from build123d import *

# Parameters (mm, degrees)
BOSS_EXTRUDE1_DEPTH                           = 15.875
BOSS_EXTRUDE2_DEPTH                           = 15.875
CBORE_FOR_1_4_SOCKET_HEAD_CAP_SCREW1_AT_COUNT = 2
CBORE_FOR_1_4_SOCKET_HEAD_CAP_SCREW1_AT_PITCH = 41.275
MOVE_FACE1_BY                                 = 0.127
MOVE_FACE1_2_BY                               = 0.127
MOVE_START                                    = 28.575
MOVE_FACE2_OUTLINE_W                          = 15.875
MOVE_FACE2_OUTLINE_H                          = 60.325
MOVE_FACE2_OUTLINE_R                          = 5.55625
MOVE_FACE2_DEPTH                              = 6.35
MOVE_START_2                                  = 22.225
MOVE_FACE2_2_OUTLINE_R                        = 5.55625
MOVE_FACE2_2_OUTLINE_R_2                      = 3.57124
MOVE_FACE2_2_DEPTH                            = 6.35


with BuildPart() as part:
    # Sketch1 → Boss-Extrude1 (new body)
    with BuildSketch(Plane(origin=(0, 0, 0), x_dir=(0, 0, -1), z_dir=(1, 0, 0))):
        with BuildLine():
            Line((30.1625, 0), (14.2875, 0))
            ThreePointArc((14.2875, 0), (0, -14.2875), (-14.2875, 0))
            Line((-14.2875, 0), (-30.1625, 0))
            Line((-30.1625, 0), (-30.1625, -34.925))
            Line((-30.1625, -34.925), (30.1625, -34.925))
            Line((30.1625, -34.925), (30.1625, 0))
        make_face()
    extrude(amount=BOSS_EXTRUDE1_DEPTH)


with BuildPart() as body_2:
    # Sketch1<3> → Boss-Extrude2 (new body)
    with BuildSketch(Plane(origin=(0, 0, 0), x_dir=(0, 0, -1), z_dir=(1, 0, 0))):
        with BuildLine():
            ThreePointArc((-14.2875, 0), (0, 14.2875), (14.2875, 0))
            Line((14.2875, 0), (30.1625, 0))
            Line((30.1625, 0), (30.1625, 34.925))
            Line((30.1625, 34.925), (-30.1625, 34.925))
            Line((-30.1625, 34.925), (-30.1625, 0))
            Line((-30.1625, 0), (-14.2875, 0))
        make_face()
    extrude(amount=BOSS_EXTRUDE2_DEPTH)


with BuildPart() as cbore_for_1_4_socket_head_cap_screw1_tool:
    # Sketch4 → CBORE for 1/4 Socket Head Cap Screw1 (revolve)
    with BuildSketch(Plane(origin=(7.9375, 34.925, 20.6375), x_dir=(0, 0, 1), z_dir=(1, 0, 0))):
        Polygon((0, 0), (0, 69.85), (3.57124, 69.85), (3.57124, 6.35), (5.55625, 6.35), (5.55625, 0.635), (6.19125, 0), align=None)
    cbore_for_1_4_socket_head_cap_screw1 = revolve(axis=Axis((7.9375, 41.275, 20.6375), (0, -1, 0)))


with BuildPart() as part_1:
    add(part.part)

    # CBORE for 1/4 Socket Head Cap Screw1: cut by cbore_for_1_4_socket_head_cap_screw1_tool
    add(cbore_for_1_4_socket_head_cap_screw1_tool.part, mode=Mode.SUBTRACT)


with BuildPart() as body_2_1:
    add(body_2.part)

    # CBORE for 1/4 Socket Head Cap Screw1: cut by cbore_for_1_4_socket_head_cap_screw1_tool
    add(cbore_for_1_4_socket_head_cap_screw1_tool.part, mode=Mode.SUBTRACT)


with BuildPart() as cbore_for_1_4_socket_head_cap_screw1_at_tool:
    # CBORE for 1/4 Socket Head Cap Screw1 at: CBORE for 1/4 Socket Head Cap Screw1 ×2
    with Locations(*[(0, 0, -i * CBORE_FOR_1_4_SOCKET_HEAD_CAP_SCREW1_AT_PITCH) for i in range(1, CBORE_FOR_1_4_SOCKET_HEAD_CAP_SCREW1_AT_COUNT)]):
        add(cbore_for_1_4_socket_head_cap_screw1)


with BuildPart() as part_2:
    add(part_1.part)

    # CBORE for 1/4 Socket Head Cap Screw1 at: cut by cbore_for_1_4_socket_head_cap_screw1_at_tool
    add(cbore_for_1_4_socket_head_cap_screw1_at_tool.part, mode=Mode.SUBTRACT)

    # Move Face1 2: a curved face moved inward by 0.127
    add(Solid.thicken(part_2.faces().sort_by_distance((7.9375, -14.2875, 0))[0], -MOVE_FACE1_2_BY), mode=Mode.SUBTRACT)

    # Chamfer2
    # the kernel refuses this chamfer: 0.635 mm, written as the material it takes off along each edge
    with BuildSketch(Plane(origin=(0, 0, 0), x_dir=(0, 0.1132288377802066, -0.9935689358544497), z_dir=(0, 0.9935689358544497, 0.1132288377802066))) as chamfer2_piece_1:
        with BuildLine():
            Line((15.067460512, 0.017960512), (14.396539488, -0.652960512))
            Line((14.396539488, -0.652960512), (14.383839488, -0.652960512))
            ThreePointArc((14.383839488, -0.652960512), (14.4018, -0.326480256), (14.4018, 0))
            Line((14.4018, 0), (14.4145, 0.0127))
            ThreePointArc((14.4145, 0.0127), (14.740980256, 0.0127), (15.067460512, 0.030660512))
            Line((15.067460512, 0.030660512), (15.067460512, 0.017960512))
        make_face()
    revolve(axis=Axis((0, 0, 0), (-1, 0, 0)), revolution_arc=193.002955297, mode=Mode.SUBTRACT)
    with BuildSketch(Plane(origin=(-1.600435701, 0, -14.4145), x_dir=(0, 0, -1), z_dir=(1, 0, 0))) as chamfer2_piece_2:
        with BuildLine():
            Line((0.639932919, 0.017577515), (-0.031172593, -0.625784266))
            Line((-0.031172593, -0.625784266), (-0.043861283, -0.625248401))
            ThreePointArc((-0.043861283, -0.625248401), (-0.016099091, -0.31288099), (-0.0127, 0))
            Line((-0.0127, 0), (0, 0.0127))
            ThreePointArc((0, 0.0127), (0.319966459, 0.0127), (0.639932919, 0.030277515))
            Line((0.639932919, 0.030277515), (0.639932919, 0.017577515))
        make_face()
    extrude(amount=19.075871403, mode=Mode.SUBTRACT)
    with BuildSketch(Plane(origin=(-1.600435701, 0, 14.4145), x_dir=(0, -0.999777333387341, -0.021101745067597762), z_dir=(1, 0, 0))) as chamfer2_piece_3:
        with BuildLine():
            Line((0.626302721, 0.017960512), (-0.031077302, -0.639419511))
            Line((-0.031077302, -0.639419511), (-0.043774474, -0.639151519))
            ThreePointArc((-0.043774474, -0.639151519), (-0.019449023, -0.319627221), (-0.012697172, 0.000267992))
            Line((-0.012697172, 0.000267992), (0.000267992, 0.012697172))
            ThreePointArc((0.000267992, 0.012697172), (0.313151041, 0.009493172), (0.626034729, 0.030657684))
            Line((0.626034729, 0.030657684), (0.626302721, 0.017960512))
        make_face()
    extrude(amount=19.075871403, mode=Mode.SUBTRACT)
    with BuildSketch(Plane(origin=(15.875, 0, 0), x_dir=(0, 0.11322883778020662, -0.9935689358544497), z_dir=(0, 0.9935689358544497, 0.11322883778020662))) as chamfer2_piece_4:
        with BuildLine():
            Line((14.396539488, 0.652960512), (15.067460512, -0.017960512))
            Line((15.067460512, -0.017960512), (15.067460512, -0.030660512))
            ThreePointArc((15.067460512, -0.030660512), (14.740980256, -0.0127), (14.4145, -0.0127))
            Line((14.4145, -0.0127), (14.4018, 0))
            ThreePointArc((14.4018, 0), (14.4018, 0.326480256), (14.383839488, 0.652960512))
            Line((14.383839488, 0.652960512), (14.396539488, 0.652960512))
        make_face()
    revolve(axis=Axis((15.875, 0, 0), (-1, 0, 0)), revolution_arc=193.002955297, mode=Mode.SUBTRACT)


with BuildPart() as body_2_2:
    add(body_2_1.part)

    # CBORE for 1/4 Socket Head Cap Screw1 at: cut by cbore_for_1_4_socket_head_cap_screw1_at_tool
    add(cbore_for_1_4_socket_head_cap_screw1_at_tool.part, mode=Mode.SUBTRACT)

    # Move Face1: a curved face moved inward by 0.127
    add(Solid.thicken(body_2_2.faces().sort_by_distance((7.9375, 14.2875, 0))[0], -MOVE_FACE1_BY), mode=Mode.SUBTRACT)

    # Move Face2: read off the stored shape, not the designer's step
    # Move Face2 outline → Move Face2 (cut)
    with BuildSketch(Plane(origin=(0, 0, 0), x_dir=(1, 0, 0), z_dir=(0, 1, 0)).offset(MOVE_START)):
        with Locations((7.9375, 0)):
            Rectangle(MOVE_FACE2_OUTLINE_W, MOVE_FACE2_OUTLINE_H)
        with Locations((7.9375, -20.6375)):
            Circle(MOVE_FACE2_OUTLINE_R, mode=Mode.SUBTRACT)
        with Locations((7.9375, 20.6375)):
            Circle(MOVE_FACE2_OUTLINE_R, mode=Mode.SUBTRACT)
    extrude(amount=MOVE_FACE2_DEPTH, mode=Mode.SUBTRACT)

    # Move Face2 2 outline → Move Face2 2 (cut)
    # profile 1 of 2: a face of its own
    with BuildSketch(Plane(origin=(0, 0, 0), x_dir=(1, 0, 0), z_dir=(0, 1, 0)).offset(MOVE_START_2)):
        with Locations((7.9375, 20.6375)):
            Circle(MOVE_FACE2_2_OUTLINE_R)
        with Locations((7.9375, 20.6375)):
            Circle(MOVE_FACE2_2_OUTLINE_R_2, mode=Mode.SUBTRACT)
    # profile 2 of 2: a face of its own
    with BuildSketch(Plane(origin=(0, 0, 0), x_dir=(1, 0, 0), z_dir=(0, 1, 0)).offset(MOVE_START_2)):
        with Locations((7.9375, -20.6375)):
            Circle(MOVE_FACE2_2_OUTLINE_R)
        with Locations((7.9375, -20.6375)):
            Circle(MOVE_FACE2_2_OUTLINE_R_2, mode=Mode.SUBTRACT)
    extrude(amount=MOVE_FACE2_2_DEPTH, mode=Mode.SUBTRACT)

    # Move Face2 3: loft between two sections, ruled curve by curve
    move_face2_3_from = [
        Edge.make_three_point_arc((7.9375, 27.94, -15.08125), (13.49375, 27.94, -20.6375), (7.9375, 27.94, -26.19375)),
        Edge.make_three_point_arc((7.9375, 27.94, -26.19375), (2.38125, 27.94, -20.6375), (7.9375, 27.94, -15.08125)),
    ]
    move_face2_3_to = [
        Edge.make_three_point_arc((7.9375, 28.575, -14.44625), (14.12875, 28.575, -20.6375), (7.9375, 28.575, -26.82875)),
        Edge.make_three_point_arc((7.9375, 28.575, -26.82875), (1.74625, 28.575, -20.6375), (7.9375, 28.575, -14.44625)),
    ]
    move_face2_3 = Solid(Shell([*[Face.make_surface_from_curves(move_face2_3_from[k], move_face2_3_to[k]) for k in range(2)], Face(Wire(move_face2_3_from)), Face(Wire(move_face2_3_to))]))
    add(move_face2_3, mode=Mode.SUBTRACT)

    # Move Face2 4: loft between two sections, ruled curve by curve
    move_face2_4_from = [
        Edge.make_three_point_arc((7.9375, 27.94, 26.19375), (13.49375, 27.94, 20.6375), (7.9375, 27.94, 15.08125)),
        Edge.make_three_point_arc((7.9375, 27.94, 15.08125), (2.38125, 27.94, 20.6375), (7.9375, 27.94, 26.19375)),
    ]
    move_face2_4_to = [
        Edge.make_three_point_arc((7.9375, 28.575, 26.82875), (14.12875, 28.575, 20.6375), (7.9375, 28.575, 14.44625)),
        Edge.make_three_point_arc((7.9375, 28.575, 14.44625), (1.74625, 28.575, 20.6375), (7.9375, 28.575, 26.82875)),
    ]
    move_face2_4 = Solid(Shell([*[Face.make_surface_from_curves(move_face2_4_from[k], move_face2_4_to[k]) for k in range(2)], Face(Wire(move_face2_4_from)), Face(Wire(move_face2_4_to))]))
    add(move_face2_4, mode=Mode.SUBTRACT)

    # Chamfer1
    # the kernel refuses this chamfer: 0.635 mm, written as the material it takes off along each edge
    with BuildSketch(Plane(origin=(0, 0, 0), x_dir=(0, -0.11322883778020673, 0.9935689358544497), z_dir=(0, -0.9935689358544497, -0.11322883778020673))) as chamfer1_piece_1:
        with BuildLine():
            Line((15.067460512, 0.017960512), (14.396539488, -0.652960512))
            Line((14.396539488, -0.652960512), (14.383839488, -0.652960512))
            ThreePointArc((14.383839488, -0.652960512), (14.4018, -0.326480256), (14.4018, 0))
            Line((14.4018, 0), (14.4145, 0.0127))
            ThreePointArc((14.4145, 0.0127), (14.740980256, 0.0127), (15.067460512, 0.030660512))
            Line((15.067460512, 0.030660512), (15.067460512, 0.017960512))
        make_face()
    revolve(axis=Axis((0, 0, 0), (-1, 0, 0)), revolution_arc=193.002955297, mode=Mode.SUBTRACT)
    with BuildSketch(Plane(origin=(-1.600435701, 0, 14.4145), x_dir=(0, 0, 1), z_dir=(1, 0, 0))) as chamfer1_piece_2:
        with BuildLine():
            Line((0.639932919, 0.017577515), (-0.031172593, -0.625784266))
            Line((-0.031172593, -0.625784266), (-0.043861283, -0.625248401))
            ThreePointArc((-0.043861283, -0.625248401), (-0.016099091, -0.31288099), (-0.0127, 0))
            Line((-0.0127, 0), (0, 0.0127))
            ThreePointArc((0, 0.0127), (0.319966459, 0.0127), (0.639932919, 0.030277515))
            Line((0.639932919, 0.030277515), (0.639932919, 0.017577515))
        make_face()
    extrude(amount=19.075871403, mode=Mode.SUBTRACT)
    with BuildSketch(Plane(origin=(-1.600435701, 0, -14.4145), x_dir=(0, 0.999777333387341, 0.021101745067597762), z_dir=(1, 0, 0))) as chamfer1_piece_3:
        with BuildLine():
            Line((0.626302721, 0.017960512), (-0.031077302, -0.639419511))
            Line((-0.031077302, -0.639419511), (-0.043774474, -0.639151519))
            ThreePointArc((-0.043774474, -0.639151519), (-0.019449023, -0.319627221), (-0.012697172, 0.000267992))
            Line((-0.012697172, 0.000267992), (0.000267992, 0.012697172))
            ThreePointArc((0.000267992, 0.012697172), (0.313151041, 0.009493172), (0.626034729, 0.030657684))
            Line((0.626034729, 0.030657684), (0.626302721, 0.017960512))
        make_face()
    extrude(amount=19.075871403, mode=Mode.SUBTRACT)
    with BuildSketch(Plane(origin=(15.875, 0, 0), x_dir=(0, -0.11322883778020675, 0.9935689358544497), z_dir=(0, -0.9935689358544497, -0.11322883778020675))) as chamfer1_piece_4:
        with BuildLine():
            Line((14.396539488, 0.652960512), (15.067460512, -0.017960512))
            Line((15.067460512, -0.017960512), (15.067460512, -0.030660512))
            ThreePointArc((15.067460512, -0.030660512), (14.740980256, -0.0127), (14.4145, -0.0127))
            Line((14.4145, -0.0127), (14.4018, 0))
            ThreePointArc((14.4018, 0), (14.4018, 0.326480256), (14.383839488, 0.652960512))
            Line((14.383839488, 0.652960512), (14.396539488, 0.652960512))
        make_face()
    revolve(axis=Axis((15.875, 0, 0), (-1, 0, 0)), revolution_arc=193.002955297, mode=Mode.SUBTRACT)


solid = body_2_2.part
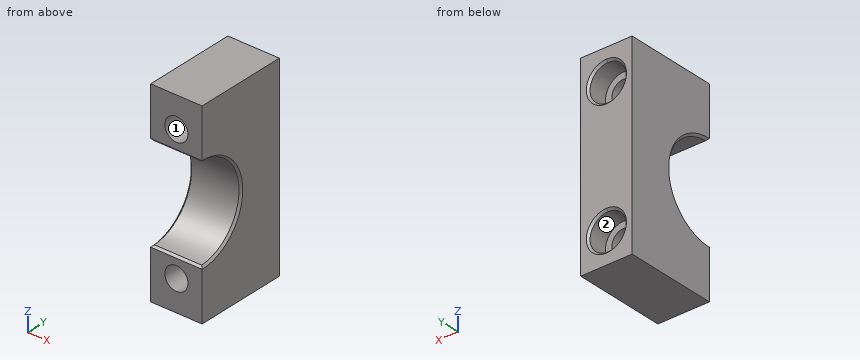
Geometry: final body of the model. Coordinates: model frame, mm. Face numbers are marked on the shaded views. A direction names the side the tool comes from. Round coordinates to 2 decimals unless told otherwise and drop trailing zeros. Loops run counter-clockwise (first coordinate to the right, second up) from the corner with the lowest first, then second, coordinate; pieces in that order, holes last. Notation, with made-up numbers: (71.25, 48.5) - (115.25, 48.5) arc R21 ccw to (115.25, 72.5) - close; hole circle Ø2 at (-26, -33.5). An arc over 180 degrees is marked (long way). Write each question's results on one line, items separated by ' | '. Start each with the question number.
1) Cut plane C-C on y = 5.25. Count the separate pieces of the cut face and the enclosed holes in it, then the cut area to 3 significant figures.
2) Access query for the marked faces 1 and 2. Directions: +Z, -Z, +X, -X, +Y, -Y. A direction counts if a zero-diameter tool reaches every point of the face in a straight line with its end or side. Return the directions, or none.
3) Line query: probe 1 along Z at (x, y) = (12.25, 22.5); probe 2 along Z at (x, y) = (8.25, 8.75); probe 3 along Z at (x, y) = (9.5, 1). Output: solid intervals per line, ascending. Write a range as [from, to].
4) Cut plane B-B on z = 0. Return loops of the section in (x, y) (1 decimal), then the cut area to 3 significant figures.
5) First-contact query: P1, Ø8, axis at x = 7.94, z = 20.64, coming from the +Y side (3 decimals). Flat tip, straight axial feed; report the tip coordinate or a pass-through.
6) Cut plane A-A on y = 21. Return loops of the section in (x, z) (1 decimal).
Verdict:
1) separate pieces: 2 | enclosed holes: 2 | area: 450 mm2
2) face 1: +Y, -Y | face 2: +Y
3) probe 1: z = [-30.16, -24.14], [-17.13, 17.13], [24.14, 30.16] | probe 2: z = [-30.16, -24.2], [-17.08, -11.45], [11.45, 17.08], [24.2, 30.16] | probe 3: z = [-30.16, -23.85], [-17.43, -14.38], [14.38, 17.43], [23.85, 30.16]
4) outline: (0, 15) - (0.6, 14.4) - (15.2, 14.4) - (15.9, 15) - (15.9, 28.6) - (0, 28.6) - close | area: 224 mm2
5) P1: stops at y = 22.225
6) outline: (0, -30.2) - (15.9, -30.2) - (15.9, 30.2) - (0, 30.2) - close; hole circle Ø7.1 at (7.9, -20.6); hole circle Ø7.1 at (7.9, 20.6)
